from build123d import *

# Parameters (mm, degrees)
SKETCH1_W           = 15
SKETCH1_H           = 7.5
BOSS_EXTRUDE1_DEPTH = 23
SKETCH10_W          = 3
SKETCH10_H          = 17
SKETCH10_W_2        = 3.5
CUT_EXTRUDE5_DEPTH  = 29.464890655
SKETCH11_R          = 2.75
CUT_EXTRUDE6_DEPTH  = 30.966648128


with BuildPart() as part:
    # Sketch1 → Boss-Extrude1 (new body)
    with BuildSketch(Plane(origin=(0, 0, 0), x_dir=(1, 0, 0), z_dir=(0, 1, 0))):
        with Locations((7.5, 3.75)):
            Rectangle(SKETCH1_W, SKETCH1_H)
    extrude(amount=BOSS_EXTRUDE1_DEPTH)

    # Mirror1: part across plane


with BuildPart() as part_1:
    add(part.part)
    add(part.part.mirror(Plane(origin=(0, 23, 0), x_dir=(1, 0, 0), z_dir=(0, 0, -1))))

    # Sketch10 → Cut-Extrude5 (cut, through all)
    with BuildSketch(Plane(origin=(15, 0, 0), x_dir=(0, 0, -1), z_dir=(1, 0, 0))):
        with Locations((-6, 11.5)):
            Rectangle(SKETCH10_W, SKETCH10_H)
        with Locations((6, 11.5)):
            Rectangle(SKETCH10_W, SKETCH10_H)
        with Locations((0, 11.5)):
            Rectangle(SKETCH10_W_2, SKETCH10_H)
    extrude(amount=-CUT_EXTRUDE5_DEPTH, mode=Mode.SUBTRACT)

    # Sketch11 → Cut-Extrude6 (cut, through all)
    with BuildSketch(Plane(origin=(0, 0, -4.5), x_dir=(-1, 0, 0), z_dir=(0, 0, -1))):
        with Locations(Location((-7.5, 11.5, 0), (0, 0, 90))):
            Circle(SKETCH11_R)
    extrude(amount=-CUT_EXTRUDE6_DEPTH, mode=Mode.SUBTRACT)


solid = part_1.part
The listing builds one solid part. Answer for the finished solid, in the listing's coordinates (mm). A direction names the side the tool comes from. Coordinates: 2 decimals unless noted, no trailing zeros. Write each loop counter-clockwise with the first axis right and the second up, starting at its lowest first coordinate (ties: lowest second). Pieces come first, ordered by that corner, then holes. Notation, with made-up numbers: M -27,25.25 L 24,25.25 A23 ccw 24,58.25 Z; hole C 68.5,-11.75 d7. An arc over 180 degrees is marked long. Put each result on its own line as item: value. Start each with the question number.
1. For a pull along Z with two mould halves and no side action, classify faces 4 (the flat face through (7, 21, -7.5)), 5 (the flat face through (11, 11, -1.75)), 6 (the flat face through (8, 3, 6)) as pulls with the +Z half, pulls with the -Z half, needs draft (parallel to the pull), parting line crosses it, or undercut.
2. Flat-ended cylindrical pins translate along their axes: P1, Ø1, axis at x = 5.5, y = 19, coming from the +Z side; P2, Ø6, axis at x = 6.5, y = 5, coming from the -Z side; P3, Ø4.5, axis at x = 9.5, y = 15.5, coming from the -Z side. Find the tip coordinate at first contact, or state that the pin passes through.
3. A cutting plane is placed at D-D on y = 11.5. Write down the section's boundary in (x, z), then the cut area to 4 significant figures.
4. A cutting plane is placed at A-A on y = 15.5. Write down the section's boundary in (x, z), then the cut area to 3 significant figures.
5. A cutting plane is placed at B-B on z = 5.5. Write down the section's boundary in (x, y), then the cut area to 3 significant figures.
6. A cutting plane is placed at C-C on x = 11.5. Write down the section's boundary in (y, z), then the cut area to 4 significant figures.
7. Consider line 1 (Y direction, x = 2.75, z = 5.5); line 2 (X direction, y = 11.5, z = -3.25); line 3 (Z direction, x = 3.5, y = 9.25). Determine where each line is inside the solid, lowest interval first. Write a range as from..to.
8. Which of the six approach directions +Z, -Z, +X, -X, +Y, -Y give full straight-line access (tool end or side, diameter ignored) to faces 1 (the flat face through (8, 3, 0)), 2 (the flat face through (11, 11, -4.5)), 3 (the flat face through (11, 11, 4.5))?
Resolved:
1. face 4: pulls with the -Z half
1. face 5: undercut
1. face 6: needs draft
2. P1: stops at z = 4.5
2. P2: stops at z = -7.5
2. P3: stops at z = -4.5
3. outline: M 0,-4.5 L 4.75,-4.5 L 4.75,-1.75 L 0,-1.75 Z; M 0,1.75 L 4.75,1.75 L 4.75,4.5 L 0,4.5 Z; M 10.25,-4.5 L 15,-4.5 L 15,-1.75 L 10.25,-1.75 Z; M 10.25,1.75 L 15,1.75 L 15,4.5 L 10.25,4.5 Z
3. area: 52.25 mm2
4. outline: M 0,-4.5 L 15,-4.5 L 15,-1.75 L 0,-1.75 Z; M 0,1.75 L 15,1.75 L 15,4.5 L 0,4.5 Z
4. area: 82.5 mm2
5. outline: M 0,0 L 15,0 L 15,3 L 0,3 Z; M 0,20 L 15,20 L 15,23 L 0,23 Z
5. area: 90.0 mm2
6. outline: M 0,-7.5 L 3,-7.5 L 3,-4.5 L 20,-4.5 L 20,-7.5 L 23,-7.5 L 23,7.5 L 20,7.5 L 20,4.5 L 3,4.5 L 3,7.5 L 0,7.5 Z; hole M 3,-1.75 L 20,-1.75 L 20,1.75 L 3,1.75 Z
6. area: 183.5 mm2
7. line 1: y = 0..3, 20..23
7. line 2: x = 0..4.75, 10.25..15
7. line 3: z = -4.5..-1.75, 1.75..4.5
8. face 1: +X, -X
8. face 2: -Z, +X, -X
8. face 3: +Z, +X, -X
